Verification items for this drawing (mm, ordinates from the low corner). Round coordinates to 2 decimals unless told otherwise and drop trailing zeros. Loops run counter-clockwise (first coordinate to the right, second up) from the corner with the lowest first, then second, coordinate; pieces in that order, holes last. Notation, with made-up numbers: M 9,80.25 L 51,80.25 A24 cw 51,99.25 Z; hole C 24.25,39.25 d8. An arc over 180 degrees is marked long. One line per item, written item: value.
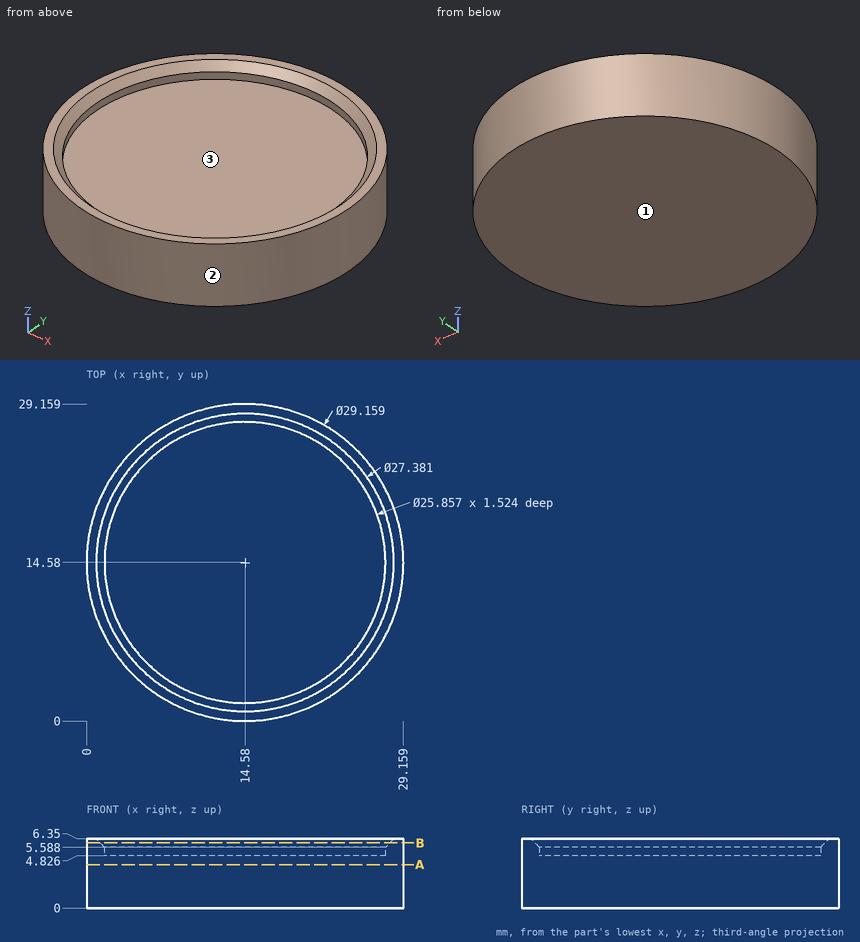
(1) Thickness scan on L1, parallel to Z at x = 2.5, y = 11.75; L2, parallel to X at y = 3.75, z = 5.5 (1 decimal); L3, parallel to Y at x = 10.5, z = 5. Record the ranges inside material, lowest first. Write a range as from..to.
Completed:
L1: z = 0..4.83
L2: x = 4.8..7.5, 21.6..24.3
L3: y = 0.58..2.31, 26.85..28.58
(2) Sectioned sample at B-B on z = 6. Enter the section's corners in (x, y), and give its area (3 significant figures).
Completed:
outline: C 14.58,14.58 d29.16; hole C 14.58,14.58 d26.68
area: 109 mm^2
(3) Sectioned sample at A-A on z = 4. Enter the section's corners in (x, y).
Completed:
outline: C 14.58,14.58 d29.16
(4) Depth check by flat-ended pin: pin 1 Ø13 at (x, y) = (16, 16) entering from +Z; pin 2 Ø2 at (y, z) = (16, 4.5) entering from +X; pin 3 Ø1 at (y, z) = (16.5, 5) entering from +X. Enter the tip coordinate at first touch or a pass-through.
Completed:
pin 1: stops at z = 4.83
pin 2: stops at x = 29.15
pin 3: stops at x = 29.09
(5) Mould release check, pull along Y, two halves, no side actions. Record for the marked faces 1, 2 and 3: +Y half, -Y half, draft (parallel to the pull), parting line (faces both ways), or undercut.
Completed:
face 1: draft
face 2: parting line
face 3: undercut
